Build history of the part. All positions in model axes, mm. A direction names the side the tool comes from. Give positions to 0.01 mm unless a question says otherwise; leave off trailing zeros. Order: outer loops, then holes, each group sorted by start corner. A loop starts at its lowest first (then second) coordinate and runs counter-clockwise, first axis right, second up. Notation, with made-up numbers: (55, 49.25) - (100, 49.25) arc R28 ccw to (100, 88.25) - close; hole circle Ø2 at (73.5, 7). An arc over 180 degrees is marked (long way). One line per item, written item: value.
Autodesk Inventor part; units mm, degrees
ref_plane "YZ Plane" through (0, 0, 0) normal (1, 0, 0) x (0, 1, 0)
ref_plane "XZ Plane" through (0, 0, 0) normal (0, 1, 0) x (-1, 0, 0)
ref_plane "XY Plane" through (0, 0, 0) normal (0, 0, 1) x (1, 0, 0)
sketch "Sketch1" plane through (0, 0, 0) normal (0, 0, 1) x (1, 0, 0)
  line L0 (-9.4869, 5.4773) -> (0, 10.9545)
  line L1 (0, 10.9545) -> (9.4869, 5.4773)
  line L2 (9.4869, 5.4773) -> (9.4869, -5.4773)
  line L3 (9.4869, -5.4773) -> (0, -10.9545)
  line L4 (0, -10.9545) -> (-9.4869, -5.4773)
  line L5 (-9.4869, -5.4773) -> (-9.4869, 5.4773)
  point P0 (0, 0)
  point P1 (0, 0)
  dimension "d0" = 18.9738
extrude "Extrusion1" add sketch "Sketch1" along normal blind 18.034
sketch "Sketch2" plane through (0, 0, 18.034) normal (0, 0, 1) x (1, 0, 0)
  circle A0 centre (0, 0) radius 12.1793
  dimension "d3" = 24.3586
extrude "Extrusion2" add sketch "Sketch2" along normal blind 1.2065
sketch "Sketch3" plane through (0, 0, 0) normal (0, 0, -1) x (-1, 0, 0)
  circle A0 centre (0, 0) radius 8.8455
  dimension "d6" = 17.6911
extrude "Extrusion3" add sketch "Sketch3" along normal blind 1.4478
sketch "Sketch4" plane through (0, 0, -1.4478) normal (0, 0, -1) x (-1, 0, 0)
  circle A0 centre (0, 0) radius 9.3663
  dimension "d9" = 18.7325
extrude "Extrusion4" add sketch "Sketch4" along normal blind 1.9939
sketch "Sketch5" plane through (0, 0, 19.2405) normal (0, 0, 1) x (1, 0, 0)
  circle A0 centre (0, 0) radius 3
  dimension "d12" = 6
extrude "Extrusion5" cut sketch "Sketch5" against normal through all
sketch "Sketch6" plane through (0, 10.9545, 18.034) normal (-0.5, 0.8660254, 0) x (0.8660254, 0.5, 0)
  line L0 (-10.9545, 0) -> (0, 0)
  line L1 (-10.9545, 18.034) -> (0, 18.034)
  circle A0 centre (-5.4773, 8.9662) radius 1.6336
  line L2 (-5.4773, 18.034) -> (-5.4773, 0)
  dimension "d16" = 9.0678
hole "Hole1" at (-4.7434, 8.2159, 9.0678) direction (0.5, -0.8660254, 0) diameter 4.6355 depth 8.89
thread "Thread1"
properties part number "T80H-SM61" material "Aluminum-6061"
(1) Drill centre lines: line 1 (Z direction, x = -9.5, y = 7); line 2 (X direction, y = 2, z = 14.25); line 3 (Y direction, x = 1.75, z = 10.5). Where is each one in solid material? Low to high.
Completed:
line 1: 18.03 to 19.24
line 2: -9.49 to -2.24, 2.24 to 9.49
line 3: -9.94 to -2.44, 2.44 to 9.94
(2) Slice it at B-B, the plane z = 13. Give the cut face in (x, y), and give its area (4 significant figures).
Completed:
outline: (-9.49, -5.48) - (0, -10.95) - (9.49, -5.48) - (9.49, 5.48) - (0, 10.95) - (-9.49, 5.48) - close; hole circle Ø6 at (0, 0)
area: 283.5 mm²
(3) Slice it at A-A, the plane y = 0. Give the cut face in (x, z).
Completed:
outline: (-12.18, 18.03) - (-9.49, 18.03) - (-9.49, 0) - (-8.85, 0) - (-8.85, -1.45) - (-9.37, -1.45) - (-9.37, -3.44) - (-3, -3.44) - (-3, 19.24) - (-12.18, 19.24) - close; (3, -3.44) - (9.37, -3.44) - (9.37, -1.45) - (8.85, -1.45) - (8.85, 0) - (9.49, 0) - (9.49, 18.03) - (12.18, 18.03) - (12.18, 19.24) - (3, 19.24) - close
(4) Pin check, flat tips, straight feed: P1, Ø9, axis at y = 1.5, z = 10, coming from the -X side; P2, Ø3, axis at y = 2, z = 5, coming from the +X side; P3, Ø6, axis at x = -2.5, z = 1, coming from the +Y side; P4, Ø3.5, axis at x = 0, y = 0, coming from the -Z side. Stop position of each tip, or through.
Completed:
P1: x = -9.49
P2: x = 9.49
P3: y = 10.95
P4: through
(5) Pull direction X, two halves, no side cores. Call faces 1 (the face through (7.02, 5.38, -0.71)), 2 (the face through (0, -9, 0)), 3 (the face through (-1.04, 5.91, 10.14)): +X half, -X half, draft (parallel to the pull), parting line (faces both ways), or undercut.
Completed:
face 1: parting line
face 2: draft
face 3: undercut
(6) 3-axis set-ups, long thin cutter, end or side, ignore diameter. For faces 4 (the face through (4, -9, 18.034)), 5 (the face through (4.677, 8.254, 8.891)), 6 (the face through (9.487, 0, 9)), 7 (the face through (-5.86, 7.57, 6.89)), 8 (the face through (-4.677, -8.254, 8.891)): which of +Z, -Z, +X, -X, +Y, -Y reach the whole face in a straight line?
Completed:
face 4: -Z
face 5: -Z, +X, +Y
face 6: -Z, +X, +Y, -Y
face 7: -Z, -X, +Y
face 8: -Z, -X, -Y
(7) Slice it at C-C, the plane x = 7.5. Give the cut face in (y, z).
Completed:
outline: (-9.6, 18.03) - (-6.62, 18.03) - (-6.62, 0) - (-4.69, 0) - (-4.69, -1.45) - (-5.61, -1.45) - (-5.61, -3.44) - (5.61, -3.44) - (5.61, -1.45) - (4.69, -1.45) - (4.69, 0) - (6.62, 0) - (6.62, 18.03) - (9.6, 18.03) - (9.6, 19.24) - (-9.6, 19.24) - close
